Here's how the part is built. I have some questions about the finished solid (model axes, mm). Coordinates: 2 decimals unless noted, no trailing zeros. Write each loop counter-clockwise with the first axis right and the second up, starting at its lowest first coordinate (ties: lowest second). Pieces come first, ordered by that corner, then holes.
(1) Imagine slicing it at A-A, the plane z = -412.75. List the corners of the cut face in (x, y) for me, plus the area to 3 significant figures.
(2) For pin 1 Ø6 at (x, z) = (84, -144) entering from +Y, with a flat end and sliding along its axis, tell me the tip position at first contact or that it passes through.
(3) Imagine slicing it at B-B, the plane x = 116.5. State how many separate pieces and enclosed holes the cut face has, plus the area to 3 significant figures.
(4) Imagine slicing it at C-C, the plane z = 206.5. List the corners of the cut face in (x, y) for me, plus the area to 3 significant figures.
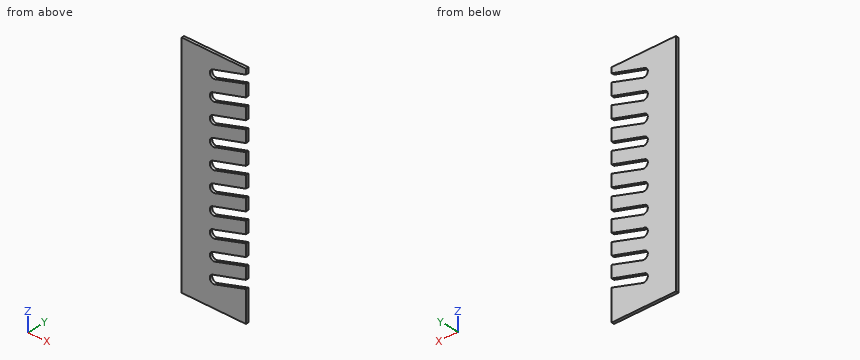
```python
from build123d import *

# Parameters (mm, degrees)
F1_DEPTH = 12.7


with BuildPart() as f1:
    # F0 (on Front) → F1 (new body)
    with BuildSketch(Plane.XZ):
        with BuildLine():
            Line((152.4, 508), (152.4, 533.4))
            Line((152.4, 533.4), (-152.4, 533.4))
            Line((-152.4, 533.4), (-152.4, -533.4))
            Line((-152.4, -533.4), (152.4, -533.4))
            Line((152.4, -533.4), (152.4, -387.35))
            Line((152.4, -387.35), (5.424796, -431.011273))
            ThreePointArc((5.424796, -431.011273), (-18.287138, -418.086955), (-5.248992, -394.43742))
            Line((-5.248992, -394.43742), (152.4, -349.25))
            Line((152.4, -349.25), (152.4, -292.1))
            Line((152.4, -292.1), (5.424796, -335.761273))
            ThreePointArc((5.424796, -335.761273), (-18.287138, -322.836955), (-5.248992, -299.18742))
            Line((-5.248992, -299.18742), (152.4, -254))
            Line((152.4, -254), (152.4, -196.85))
            Line((152.4, -196.85), (5.424796, -240.511273))
            ThreePointArc((5.424796, -240.511273), (-16.775419, -231.277061), (-12.251628, -207.66233))
            ThreePointArc((-12.251628, -207.66233), (-5.424796, -203.988727), (2.300448, -203.339409))
            Line((2.300448, -203.339409), (152.4, -158.75))
            Line((152.4, -158.75), (152.4, -101.6))
            Line((152.4, -101.6), (5.424796, -145.261273))
            ThreePointArc((5.424796, -145.261273), (-18.287138, -132.336955), (-5.248992, -108.68742))
            Line((-5.248992, -108.68742), (152.4, -63.5))
            Line((152.4, -63.5), (152.4, -6.35))
            Line((152.4, -6.35), (5.424796, -50.011273))
            ThreePointArc((5.424796, -50.011273), (-18.287138, -37.086955), (-5.248992, -13.43742))
            Line((-5.248992, -13.43742), (152.4, 31.75))
            Line((152.4, 31.75), (152.4, 88.9))
            Line((152.4, 88.9), (5.424796, 45.238727))
            ThreePointArc((5.424796, 45.238727), (-18.287138, 58.163045), (-5.248992, 81.81258))
            Line((-5.248992, 81.81258), (152.4, 127))
            Line((152.4, 127), (152.4, 184.15))
            Line((152.4, 184.15), (11.907693, 143.880254))
            ThreePointArc((11.907693, 143.880254), (5.248992, 140.43742), (-2.222457, 139.830085))
            ThreePointArc((-2.222457, 139.830085), (-18.987372, 157.206565), (-5.248992, 177.06258))
            Line((-5.248992, 177.06258), (152.4, 222.25))
            Line((152.4, 222.25), (152.4, 279.4))
            Line((152.4, 279.4), (5.424796, 235.738727))
            ThreePointArc((5.424796, 235.738727), (-18.287138, 248.663045), (-5.248992, 272.31258))
            Line((-5.248992, 272.31258), (152.4, 317.5))
            Line((152.4, 317.5), (152.4, 374.65))
            Line((152.4, 374.65), (5.424796, 330.988727))
            ThreePointArc((5.424796, 330.988727), (-18.287138, 343.913045), (-5.248992, 367.56258))
            Line((-5.248992, 367.56258), (152.4, 412.75))
            Line((152.4, 412.75), (152.4, 469.9))
            Line((152.4, 469.9), (5.424796, 426.238727))
            ThreePointArc((5.424796, 426.238727), (-18.287138, 439.163045), (-5.248992, 462.81258))
            Line((-5.248992, 462.81258), (152.4, 508))
        make_face()
    extrude(amount=F1_DEPTH)


solid = f1.part
```
Recorded:
1. outline: (-152.4, -12.7) - (-19.05, -12.7) - (-19.05, 0) - (-152.4, 0) - close; (66.9, -12.7) - (152.4, -12.7) - (152.4, 0) - (66.9, 0) - close
1. area: 2,780 mm2
2. pin 1: stops at y = 0
3. separate pieces: 11
3. enclosed holes: 0
3. area: 8,670 mm2
4. outline: (-152.4, -12.7) - (97.45, -12.7) - (97.45, 0) - (-152.4, 0) - close
4. area: 3,170 mm2
